The listing builds one solid part. Answer for the finished solid, in the listing's coordinates (mm). A direction names the side the tool comes from. Give positions to 0.01 mm unless a question says otherwise; leave off trailing zeros. Order: outer loops, then holes, each group sorted by start corner. A loop starts at its lowest first (then second) coordinate and runs counter-clockwise, first axis right, second up. Notation, with made-up numbers: (-12, 75) - (-7, 75) arc R11 ccw to (-7, 82) - close; hole circle Ø3 at (81.5, -0.75). An arc over 180 degrees is marked (long way). Write each question's results on one line, items separated by ' | '. Start each with the question number.
1. Flat-ended cylindrical pins translate along their axes: pin 1 (0.5 mm diameter, centred on y = -0.5, z = 1, fed in from +X); pin 2 (0.5 mm diameter, centred on x = 0.5, y = -0.5, fed in from -Z); pin 3 (0.8 mm diameter, centred on x = -1, y = -0.5, fed in from +Z). Find the tip coordinate at first contact, or state that the pin passes through.
2. Section B-B (y = -5.75) is taken. Give the vertices of the cut face in (x, z), and give its area (3 significant figures).
3. Section A-A (y = -1.75) is taken. Give the vertices of the cut face in (x, z), and give its area (3 significant figures).
4. Find the intervals of material crossed by L1, parallel to Y at x = 1.05, z = 0.95; L2, parallel to Y at x = 0.15, z = -0.5; L3, parallel to Z at x = 1, y = -12, in increasing order.
5. Determine the mould class of faces 1 (the face through (1, -2.5, 1)), 2 (the face through (0.9, -0.5, 0.45)), 3 (the face through (0.27, -8.17, 1.22)) for opening direction Z: released by +Z, released by -Z, zero draft, split by the parting line, or undercut.
6. Which of the six approach directions +Z, -Z, +X, -X, +Y, -Y give full straight-line access (tool end or side, diameter ignored) to faces 4 (the face through (-1.29, -1.587, -2.024)), 5 (the face through (0, -0.6, -1.4))?
from build123d import *

# Parameters (mm, degrees)
CUT_EXTRUDE1_DEPTH = 1


with BuildPart() as part:
    # Sketch2 → Revolve1 (revolve)
    with BuildSketch(Plane.XY):
        with BuildLine():
            Line((-2.4, -2.5), (-2.4, -0.7))
            add(Edge.make_bspline(
                [(0, 0), (-2.4, 0), (-2.4, -0.7)],
                knots=[4.71238898, 4.71238898, 4.71238898, 6.283185307, 6.283185307, 6.283185307], degree=2, weights=[1, 0.707106781, 1]))
            Line((0, 0), (0, -14.5))
            Line((0, -14.5), (-0.75, -14.5))
            Line((-0.75, -14.5), (-1.25, -14))
            Line((-1.25, -14), (-1.25, -2.5))
            Line((-1.25, -2.5), (-2.4, -2.5))
        make_face()
    revolve(axis=Axis((0, 0, 0), (0, -1, 0)))

    # Sketch3 → Cut-Extrude1 (cut)
    with BuildSketch(Plane(origin=(0, 0, 0), x_dir=(1, 0, 0), z_dir=(0, 1, 0))):
        Polygon((-0.45, 1.4), (0.45, 1.4), (0.45, 0.45), (1.4, 0.45), (1.4, -0.45), (0.45, -0.45), (0.45, -1.4), (-0.45, -1.4), (-0.45, -0.45), (-1.4, -0.45), (-1.4, 0.45), (-0.45, 0.45), align=None)
    extrude(amount=-CUT_EXTRUDE1_DEPTH, mode=Mode.SUBTRACT)


solid = part.part
Reported:
1) pin 1: x = 2.26 | pin 2: z = -2.38 | pin 3: z = 2.31
2) outline: circle Ø2.5 at (0, 0) | area: 4.91 mm²
3) outline: circle Ø4.8 at (0, 0) | area: 18.1 mm²
4) L1: -2.5 to -0.13 | L2: -14.5 to -1 | L3: -0.75 to 0.75
5) face 1: zero draft | face 2: undercut | face 3: split by the parting line
6) face 4: +Y, -Y | face 5: +Y
